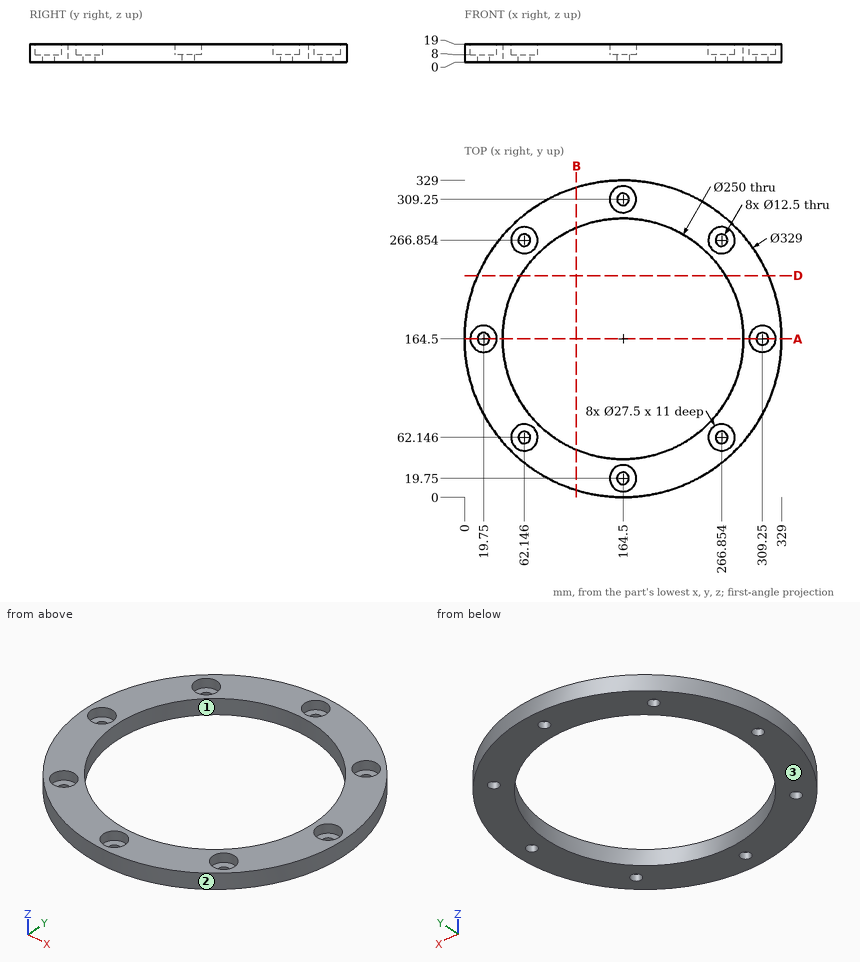
Geometry check sheet. Reference: drawing and pictorial views, mm from the part's lowest x, y, z. Round coordinates to 2 decimals unless told otherwise and drop trailing zeros. Order: outer loops, then holes, each group sorted by start corner. A loop starts at its lowest first (then second) coordinate and runs counter-clockwise, first axis right, second up. Notation, with made-up numbers: (26, 37.25) - (80, 37.25) arc R13 ccw to (80, 62.25) - close; hole circle Ø10 at (82, 37.5). An arc over 180 degrees is marked (long way). Write item = value, one per line.
Q1. Section check A-A (y = 164.5). Record the boundary of the cut face in (x, z), and give its area (3 significant figures).
Computed:
outline = (0, 0) - (13.5, 0) - (13.5, 8) - (6, 8) - (6, 19) - (0, 19) - close; (26, 0) - (39.5, 0) - (39.5, 19) - (33.5, 19) - (33.5, 8) - (26, 8) - close; (289.5, 0) - (303, 0) - (303, 8) - (295.5, 8) - (295.5, 19) - (289.5, 19) - close; (315.5, 0) - (329, 0) - (329, 19) - (323, 19) - (323, 8) - (315.5, 8) - close
area = 696 mm^2
Q2. Draft check along Y on the marked faces 1, 2 and 3. Enter one of: pulls with the +Y half, pulls with the -Y half, needs draft (parallel to the pull), parting line crosses it, or undercut.
Computed:
face_1 = undercut
face_2 = parting line crosses it
face_3 = needs draft
Q3. Thickness scan on line 1 along X through (y, z) = (164.5, 5); line 2 along X through (y, z) = (164.5, 12). Record the ranges inside material, lowest first.
Computed:
line_1 = 0 to 13.5, 26 to 39.5, 289.5 to 303, 315.5 to 329
line_2 = 0 to 6, 33.5 to 39.5, 289.5 to 295.5, 323 to 329
Q4. Go/stop test with flat-tipped pins: pin 1 (2 mm diameter, centred on x = 151, z = 10, fed in from -Y); pin 2 (1 mm diameter, centred on x = 233, z = 5, fed in from +Y); pin 3 (8 mm diameter, centred on x = 65, y = 262.5, fed in from +Z). Record where each tip stops, or that it passes through.
Computed:
pin_1 = 0.48
pin_2 = 314.29
pin_3 = 8
Q5. Section check D-D (y = 230). Record the boundary of the cut face in (x, z) (1 decimal).
Computed:
outline = (13.6, 0) - (58, 0) - (58, 19) - (13.6, 19) - close; (271, 0) - (315.4, 0) - (315.4, 19) - (271, 19) - close
Q6. Section check B-B (x = 116). Record the boundary of the cut face in (y, z), and give its area (3 significant figures).
Computed:
outline = (7.31, 0) - (49.29, 0) - (49.29, 19) - (7.31, 19) - close; (279.71, 0) - (321.69, 0) - (321.69, 19) - (279.71, 19) - close
area = 1,600 mm^2
